```python
from build123d import *

# Parameters (mm, degrees)
ESQUISSE1_W                       = 48
ESQUISSE1_H                       = 42.3
BOSS_EXTRU_1_DEPTH                = 42.3
DIAM_TRE_DU_PER_AGE_3_0_3_1_D     = 3
DIAM_TRE_DU_PER_AGE_3_0_3_1_DEPTH = 5


with BuildPart() as part:
    # Esquisse1 → Boss.-Extru.1 (new body)
    with BuildSketch(Plane(origin=(21.15, 0, 0), x_dir=(0, 0, -1), z_dir=(1, 0, 0))):
        with Locations((24, 0)):
            Rectangle(ESQUISSE1_W, ESQUISSE1_H)
    extrude(amount=-BOSS_EXTRU_1_DEPTH)

    # Esquisse2 → Révolution1 (revolve)
    with BuildSketch(Plane(origin=(0, 0, 0), x_dir=(1, 0, 0), z_dir=(0, 1, 0))):
        Polygon((11, 0), (0, 0), (0, -22), (2.5, -22), (2.5, -2), (11, -2), align=None)
    revolve(axis=Axis((0, 0, 0), (0, 0, 1)))

    # Diamètre du perçage Ø3.0 (3)1
    with Locations(Plane.XY):
        with Locations((15.5, 15.5), (15.5, -15.5), (-15.5, 15.5), (-15.5, -15.5)):
            Hole(DIAM_TRE_DU_PER_AGE_3_0_3_1_D / 2, depth=DIAM_TRE_DU_PER_AGE_3_0_3_1_DEPTH)


solid = part.part
```
CAD build for the part. Positions are in the model's coordinates, mm. A direction names the side the tool comes from. Coordinates: 2 decimals unless noted, no trailing zeros. Loops run counter-clockwise (first coordinate to the right, second up) from the corner with the lowest first, then second, coordinate; pieces in that order, holes last. Notation, with made-up numbers: (8.5, 26) - (29.5, 26) arc R21 cw to (29.5, 56) - close; hole circle Ø5 at (79, 54.25). An arc over 180 degrees is marked (long way). Return JSON: item names as keys, results as strings.
1. Band-saw the part on C-C (z = 16). Give the cut face in (x, y), and give its area (3 significant figures).
Result:
{"outline": "circle Ø5 at (0, 0)", "area": "19.6 mm2"}
2. Band-saw the part on A-A (x = -15.5). Give the cut face in (y, z).
Result:
{"outline": "(-21.15, -48) - (21.15, -48) - (21.15, 0) - (17, 0) - (17, -5) - (14, -5) - (14, 0) - (-14, 0) - (-14, -5) - (-17, -5) - (-17, 0) - (-21.15, 0) - close"}
3. Drop a flat-ended pin along its axis: pin 1 (1.5 mm diameter, centred on x = -15, y = 15, fed in from +Z). Give the stop position or say it passes through.
Result:
{"pin 1": "stops at z = -5"}
4. Probe L1, parallel to Y at x = -15.5, z = -1.2; L2, parallel to Y at x = -15, z = -2; L3, parallel to Z at x = -13, y = -9. List the from-to ranges inside material, lowest first. Write a range as from..to.
Result:
{"L1": "y = -21.15..-17, -14..14, 17..21.15", "L2": "y = -21.15..-16.91, -14.09..14.09, 16.91..21.15", "L3": "z = -48..0"}
5. Mould opens along Y. For faces 1 (the cylindrical face through (-14, 15.57, -2.54)), 2 (the flat face through (0, 0, 22)), 3 (the flat face through (0, -21.15, -24)) say: released by +Y, released by -Y, zero draft, split by the parting line, or undercut.
Result:
{"face 1": "undercut", "face 2": "zero draft", "face 3": "released by -Y"}
6. Band-saw the part on D-D (x = -8). Give the cut face in (y, z), and give its area (3 significant figures).
Result:
{"outline": "(-21.15, -48) - (21.15, -48) - (21.15, 0) - (7.55, 0) - (7.55, 2) - (-7.55, 2) - (-7.55, 0) - (-21.15, 0) - close", "area": "2,060 mm2"}
7. 3-axis set-ups, long thin cutter, end or side, ignore diameter. For faces 4 (the flat face through (16, -15, -5)), 5 (the flat face through (-21.15, 0, -24)): which of +Z, -Z, +X, -X, +Y, -Y reach the whole face in a straight line?
Result:
{"face 4": "+Z", "face 5": "+Z, -Z, -X, +Y, -Y"}
